from build123d import *

# Parameters (mm, degrees)
SKETCH1_W           = 16
SKETCH1_H           = 13.02
SKETCH1_W_2         = 7
BOSS_EXTRUDE1_DEPTH = 10
SKETCH1_3_W         = 16
SKETCH1_3_H         = 13.02
BOSS_EXTRUDE2_DEPTH = 2
BOSS_EXTRUDE3_DEPTH = 5
SKETCH2_R           = 1.7
CUT_EXTRUDE1_DEPTH  = 22.01
SKETCH2_3_R         = 5
SKETCH2_3_R_2       = 1.7
CUT_EXTRUDE2_DEPTH  = 2


with BuildPart() as part:
    # Sketch1 → Boss-Extrude1 (new body)
    with BuildSketch(Plane(origin=(0, 0, 0), x_dir=(1, 0, 0), z_dir=(0, 1, 0))):
        Polygon((-15, -6.51), (-15, -8.51), (15, -8.51), (15, -6.51), (8, -6.51), (-8, -6.51), align=None)
        Rectangle(SKETCH1_W, SKETCH1_H)
        Polygon((-15, 8.51), (-15, 6.51), (-8, 6.51), (8, 6.51), (15, 6.51), (15, 8.51), align=None)
        with Locations((11.5, 0)):
            Rectangle(SKETCH1_W_2, SKETCH1_H)
        with Locations((-11.5, 0)):
            Rectangle(SKETCH1_W_2, SKETCH1_H)
    extrude(amount=-BOSS_EXTRUDE1_DEPTH)

    # Sketch1<3> → Boss-Extrude2 (add)
    with BuildSketch(Plane(origin=(0, 0, 0), x_dir=(1, 0, 0), z_dir=(0, 1, 0))):
        Rectangle(SKETCH1_3_W, SKETCH1_3_H)
    extrude(amount=BOSS_EXTRUDE2_DEPTH)

    # Sketch1<4> → Boss-Extrude3 (add)
    with BuildSketch(Plane(origin=(0, 0, 0), x_dir=(1, 0, 0), z_dir=(0, 1, 0))):
        Polygon((-15, -6.51), (-15, -8.51), (15, -8.51), (15, -6.51), (8, -6.51), (-8, -6.51), align=None)
        Polygon((-15, 8.51), (-15, 6.51), (-8, 6.51), (8, 6.51), (15, 6.51), (15, 8.51), align=None)
    extrude(amount=BOSS_EXTRUDE3_DEPTH)

    # Sketch2 → Cut-Extrude1 (cut, through all)
    with BuildSketch(Plane(origin=(0, 2, 0), x_dir=(1, 0, 0), z_dir=(0, 1, 0))):
        with Locations(Location((0, 0, 0), (0, 0, 270))):
            Circle(SKETCH2_R)
    extrude(amount=-CUT_EXTRUDE1_DEPTH, mode=Mode.SUBTRACT)

    # Sketch2<3> → Cut-Extrude2 (cut)
    with BuildSketch(Plane(origin=(0, 2, 0), x_dir=(1, 0, 0), z_dir=(0, 1, 0))):
        with Locations(Location((0, 0, 0), (0, 0, 270))):
            Circle(SKETCH2_3_R)
        with Locations(Location((0, 0, 0), (0, 0, 270))):
            Circle(SKETCH2_3_R_2, mode=Mode.SUBTRACT)
    extrude(amount=-CUT_EXTRUDE2_DEPTH, mode=Mode.SUBTRACT)


solid = part.part
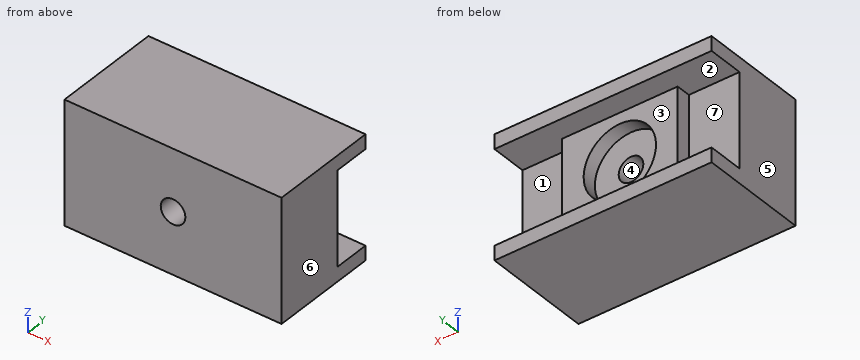
Build history of the part. All positions in model axes, mm. Face numbers are marked on the shaded views. A direction names the side the tool comes from. Round coordinates to 2 decimals unless told otherwise and drop trailing zeros. Write each loop counter-clockwise with the first axis right and the second up, starting at its lowest first coordinate (ties: lowest second). Pieces come first, ordered by that corner, then holes. Notation, with made-up numbers: M 2,70 L 45,70 A10 cw 45,83 Z; hole C -23.5,10.25 d11. An arc over 180 degrees is marked long. Answer in a Markdown table with one row per item.
1. Which spindle directions (+Z, -Z, +X, -X, +Y, -Y) get a long thin tool onto all of the face, cutting with end or side? Do the marked faces 1, 2 and 3. Say none if no direction does.
Geometry check:
| item | result |
|---|---|
| face 1 | +X, +Y |
| face 2 | +Y |
| face 3 | +X, -X, +Y |
2. Probe L1, parallel to X at y = -6.5, z = 0; L2, parallel to Z at x = 12, y = 3.75; L3, parallel to X at y = 0.5, z = 0. List the from-to ranges inside material, lowest first. Write a range as [from, to].
Geometry check:
| item | result |
|---|---|
| L1 | [-15, -1.7], [1.7, 15] |
| L2 | [-8.51, -6.51], [6.51, 8.51] |
| L3 | [-8, -5], [5, 8] |
3. Saw through at D-D (x = 11.25). List the corners of the cut face in (y, z), and give its area (3 significant figures).
Geometry check:
| item | result |
|---|---|
| outline | M -10,-8.51 L 5,-8.51 L 5,-6.51 L 0,-6.51 L 0,6.51 L 5,6.51 L 5,8.51 L -10,8.51 Z |
| area | 190 mm2 |
4. Saw through at B-B (z = 0). List the corners of the cut face in (x, y).
Geometry check:
| item | result |
|---|---|
| outline | M -15,-10 L -1.7,-10 L -1.7,0 L -5,0 L -5,2 L -8,2 L -8,0 L -15,0 Z; M 1.7,-10 L 15,-10 L 15,0 L 8,0 L 8,2 L 5,2 L 5,0 L 1.7,0 Z |
5. Saw through at A-A (y = 1.5). List the corners of the cut face in (x, z), and give its area (3 significant figures).
Geometry check:
| item | result |
|---|---|
| outline | M -15,-8.51 L 15,-8.51 L 15,-6.51 L 8,-6.51 L 8,6.51 L 15,6.51 L 15,8.51 L -15,8.51 L -15,6.51 L -8,6.51 L -8,-6.51 L -15,-6.51 Z; hole C 0,0 d10 |
| area | 250 mm2 |
6. Saw through at C-C (x = 0). List the corners of the cut face in (y, z).
Geometry check:
| item | result |
|---|---|
| outline | M -10,-8.51 L 5,-8.51 L 5,-6.51 L 2,-6.51 L 2,-5 L 0,-5 L 0,-1.7 L -10,-1.7 Z; M -10,1.7 L 0,1.7 L 0,5 L 2,5 L 2,6.51 L 5,6.51 L 5,8.51 L -10,8.51 Z |
7. Mould opens along X. For the marked faces 4, 5, 6 and 7 say: +X half, -X half, draft (parallel to the pull), parting line (faces both ways), or undercut.
Geometry check:
| item | result |
|---|---|
| face 4 | undercut |
| face 5 | -X half |
| face 6 | +X half |
| face 7 | draft |
8. Flat gauge pins, fed straight in: P1, Ø2, axis at x = -11.5, z = -3, coming from the +Y side; P2, Ø6.5, axis at x = -1, z = 2.5, coming from the +Y side; P3, Ø1.5, axis at y = 2, z = 2, coming from the -X side. Where does each tip first touch, or does it go through?
Geometry check:
| item | result |
|---|---|
| P1 | y = 0 |
| P2 | y = 2 |
| P3 | x = -8 |
